from build123d import *

# Parameters (mm, degrees)
EXTRUDE_2_DEPTH = 1


with BuildPart() as part:
    # Эскиз1 → Бобышка-Вытянуть2 (new body)
    with BuildSketch(Plane.XY):
        with BuildLine():
            Line((-152.649098001, -86.991869919), (-152.649098001, 163.008130081))
            ThreePointArc((-152.649098001, 163.008130081), (-130.68210659, 216.04113867), (-77.649098001, 238.008130081))
            Line((-77.649098001, 238.008130081), (222.350901999, 238.008130081))
            ThreePointArc((222.350901999, 238.008130081), (275.383910588, 216.04113867), (297.350901999, 163.008130081))
            Line((297.350901999, 163.008130081), (297.350901999, -86.991869919))
            Line((297.350901999, -86.991869919), (272.350901999, -86.991869919))
            Line((272.350901999, -86.991869919), (-152.649098001, -86.991869919))
        make_face()
    extrude(amount=EXTRUDE_2_DEPTH)


solid = part.part
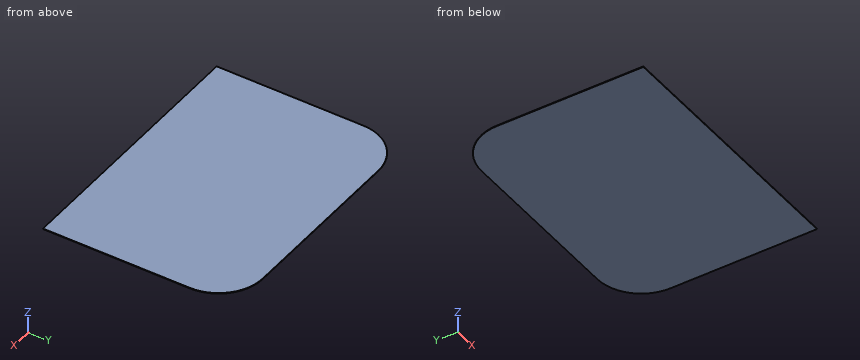
Check sheet for the modelled part. Datum: model origin and axes. Units: mm. Give positions to 0.01 mm unless a question says otherwise; leave off trailing zeros. Write each loop counter-clockwise with the first axis right and the second up, starting at its lowest first coordinate (ties: lowest second). Pieces come first, ordered by that corner, then holes. Notation, with made-up numbers: (50, 7.25) -> (56, 7.25) arc R31 cw to (56, 37.25) -> close; hole circle Ø9 at (-30.75, -26). An arc over 180 degrees is marked (long way). One line per item, written item: value. Start each with the question number.
Item 1: Section check B-B on x = -104.5. Record the cut outline in (y, z).
Item 2: Section check C-C on y = 215.5. Record the cut outline in (x, z), then the cut area to 3 significant figures.
Item 3: Section check A-A on z = 0.6. Record the cut outline in (x, y).
Item 4: Material ranges on probe 1 along X at (y, z) = (185, 0.25); probe 2 along X at (y, z) = (190.5, 0.25), recorded low to high. Write a range as from..to.
Results list:
1. outline: (-86.99, 0) -> (233.04, 0) -> (233.04, 1) -> (-86.99, 1) -> close
2. outline: (-131.22, 0) -> (275.92, 0) -> (275.92, 1) -> (-131.22, 1) -> close
2. area: 407 mm²
3. outline: (-152.65, -86.99) -> (297.35, -86.99) -> (297.35, 163.01) arc R75 ccw to (222.35, 238.01) -> (-77.65, 238.01) arc R75 ccw to (-152.65, 163.01) -> close
4. probe 1: -149.35..294.05
4. probe 2: -147.43..292.13
